Build history of the part. All positions in model axes, mm. A direction names the side the tool comes from. Round coordinates to 2 decimals unless told otherwise and drop trailing zeros. Write each loop counter-clockwise with the first axis right and the second up, starting at its lowest first coordinate (ties: lowest second). Pieces come first, ordered by that corner, then holes. Notation, with made-up numbers: (45.5, 41.25) - (92.5, 41.25) arc R15 ccw to (92.5, 55.25) - close; hole circle Ø2 at (25, 20.25). An arc over 180 degrees is marked (long way). Write each question's results on one line, items separated by ' | '.
from build123d import *

# Parameters (mm, degrees)
SKETCH_2_W                    = 30
SKETCH_2_H                    = 30
EXTRUDE_1_DEPTH               = 10
SHELL_1_T                     = -2
CUT_EXTRUDE_1_REACH           = 34.104
SKETCH_3_W                    = 28
SKETCH_3_H                    = 26
EXTRUDE_2_DEPTH               = 30
CUT_EXTRUDE_2_DEPTH           = 34.566112599
SKETCH_6_R                    = 2.375
EXTRUDE_3_DEPTH               = 1
SKETCH_7_R                    = 1
CUT_EXTRUDE_3_DEPTH           = 3
CUT_EXTRUDE_3_DRAFT           = -2
CUT_EXTRUDE_3_PROFILE_2_DEPTH = 3
CUT_EXTRUDE_3_PROFILE_2_DRAFT = -2
CUT_EXTRUDE_3_PROFILE_3_DEPTH = 3
CUT_EXTRUDE_3_PROFILE_3_DRAFT = -2
CUT_EXTRUDE_3_PROFILE_4_DEPTH = 3
CUT_EXTRUDE_3_PROFILE_4_DRAFT = -2
FILLET_2_R                    = 2
FILLET_3_R                    = 4
SKETCH_8_R                    = 1.05
CUT_EXTRUDE_4_DEPTH           = 38.710498044
CHAMFER_1_SIZE                = 1
CHAMFER_2_SIZE                = 2.001261587
CHAMFER_2_SIZE_2              = 2


with BuildPart() as part:
    # 草图2 → 凸台-拉伸1 (new body)
    with BuildSketch(Plane.XY):
        with Locations((3.057614324, -9.588661073)):
            Rectangle(SKETCH_2_W, SKETCH_2_H)
    extrude(amount=-EXTRUDE_1_DEPTH)

    # 抽壳1
    shell_1_openings = [part.faces().sort_by_distance(p)[0] for p in [
        (-11.942385676, -9.588661073, -5),
    ]]
    offset(amount=SHELL_1_T, openings=shell_1_openings, kind=Kind.INTERSECTION)

    # 草图3 → 切除-拉伸1 (cut, up to next)
    with BuildSketch(Plane.XY, mode=Mode.PRIVATE) as cut_extrude_1_sk1:
        with Locations((2.057614324, -9.588661073)):
            Rectangle(SKETCH_3_W, SKETCH_3_H)
    cut_extrude_1_tool1 = extrude(cut_extrude_1_sk1.sketch, amount=-CUT_EXTRUDE_1_REACH, mode=Mode.PRIVATE) & part.part
    add(cut_extrude_1_tool1.solids().sort_by_distance((2.057614, -9.588661, 0))[0], mode=Mode.SUBTRACT)

    # 草图4 → 凸台-拉伸2 (add)
    with BuildSketch(Plane.XZ.offset(24.588661073)):
        with BuildLine():
            Line((-11.942385676, -10), (-11.942385676, -14))
            add(Edge.make_bspline(
                [(-11.942385676, -14), (-1.471769767, -14.006598556), (8.440678476, -13.813297469), (18.057614324, -10)],
                knots=[0, 0, 0, 0, 1, 1, 1, 1], degree=3))
            Line((18.057614324, -10), (-11.942385676, -10))
        make_face()
    extrude(amount=-EXTRUDE_2_DEPTH)

    # 草图5 → 切除-拉伸2 (cut, through all)
    with BuildSketch(Plane.XY):
        with BuildLine():
            Line((6.557614324, -3.588661073), (-11.942385676, -3.588661073))
            Line((-11.942385676, -3.588661073), (-11.942385676, -15.588661073))
            Line((-11.942385676, -15.588661073), (6.557614324, -15.588661073))
            ThreePointArc((6.557614324, -15.588661073), (7.618274496, -15.149321245), (8.057614324, -14.088661073))
            Line((8.057614324, -14.088661073), (8.057614324, -5.088661073))
            ThreePointArc((8.057614324, -5.088661073), (7.618274496, -4.028000901), (6.557614324, -3.588661073))
        make_face()
    extrude(amount=-CUT_EXTRUDE_2_DEPTH, mode=Mode.SUBTRACT)

    # 草图6 → 凸台-拉伸3 (add)
    with BuildSketch(Plane.XY.offset(-8)):
        with Locations(Location((1.557614324, 0.908700453, 0), (0, 0, 180))):
            Circle(SKETCH_6_R)
        with Locations((14.057614324, 0.908700453)):
            Circle(SKETCH_6_R)
        with Locations(Location((1.557614324, -20.091299547, 0), (0, 0, 180))):
            Circle(SKETCH_6_R)
        with Locations((14.057614324, -20.091299547)):
            Circle(SKETCH_6_R)
    extrude(amount=EXTRUDE_3_DEPTH)


with BuildPart() as cut_extrude_3_tool:
    # 草图7 → 切除-拉伸3 (with draft: the straight prism first)
    with BuildSketch(Plane.XY.offset(-7)):
        with Locations((1.557614324, -20.091299547)):
            Circle(SKETCH_7_R)
    extrude(amount=-CUT_EXTRUDE_3_DEPTH)
    # 切除-拉伸3: the draft: its side faces are tilted about the plane it starts from
    cut_extrude_3_sides = [cut_extrude_3_tool.faces().sort_by_distance(p)[0] for p in [
        (0.557614324, -20.091299547, -8.5),
    ]]
    draft(cut_extrude_3_sides, Plane.XY.offset(-7), CUT_EXTRUDE_3_DRAFT)


with BuildPart() as part_1:
    add(part.part)

    # 切除-拉伸3: cut by cut_extrude_3_tool
    add(cut_extrude_3_tool.part, mode=Mode.SUBTRACT)


with BuildPart() as cut_extrude_3_profile_2_tool:
    # 草图7 → 切除-拉伸3 profile 2 (with draft: the straight prism first)
    with BuildSketch(Plane.XY.offset(-7)):
        with Locations((14.057614324, -20.091299547)):
            Circle(SKETCH_7_R)
    extrude(amount=-CUT_EXTRUDE_3_PROFILE_2_DEPTH)
    # 切除-拉伸3 profile 2: the draft: its side faces are tilted about the plane it starts from
    cut_extrude_3_profile_2_sides = [cut_extrude_3_profile_2_tool.faces().sort_by_distance(p)[0] for p in [
        (13.057614324, -20.091299547, -8.5),
    ]]
    draft(cut_extrude_3_profile_2_sides, Plane.XY.offset(-7), CUT_EXTRUDE_3_PROFILE_2_DRAFT)


with BuildPart() as part_2:
    add(part_1.part)

    # 切除-拉伸3 profile 2: cut by cut_extrude_3_profile_2_tool
    add(cut_extrude_3_profile_2_tool.part, mode=Mode.SUBTRACT)


with BuildPart() as cut_extrude_3_profile_3_tool:
    # 草图7 → 切除-拉伸3 profile 3 (with draft: the straight prism first)
    with BuildSketch(Plane.XY.offset(-7)):
        with Locations((1.557614324, 0.908700453)):
            Circle(SKETCH_7_R)
    extrude(amount=-CUT_EXTRUDE_3_PROFILE_3_DEPTH)
    # 切除-拉伸3 profile 3: the draft: its side faces are tilted about the plane it starts from
    cut_extrude_3_profile_3_sides = [cut_extrude_3_profile_3_tool.faces().sort_by_distance(p)[0] for p in [
        (0.557614324, 0.908700453, -8.5),
    ]]
    draft(cut_extrude_3_profile_3_sides, Plane.XY.offset(-7), CUT_EXTRUDE_3_PROFILE_3_DRAFT)


with BuildPart() as part_3:
    add(part_2.part)

    # 切除-拉伸3 profile 3: cut by cut_extrude_3_profile_3_tool
    add(cut_extrude_3_profile_3_tool.part, mode=Mode.SUBTRACT)


with BuildPart() as cut_extrude_3_profile_4_tool:
    # 草图7 → 切除-拉伸3 profile 4 (with draft: the straight prism first)
    with BuildSketch(Plane.XY.offset(-7)):
        with Locations((14.057614324, 0.908700453)):
            Circle(SKETCH_7_R)
    extrude(amount=-CUT_EXTRUDE_3_PROFILE_4_DEPTH)
    # 切除-拉伸3 profile 4: the draft: its side faces are tilted about the plane it starts from
    cut_extrude_3_profile_4_sides = [cut_extrude_3_profile_4_tool.faces().sort_by_distance(p)[0] for p in [
        (13.057614324, 0.908700453, -8.5),
    ]]
    draft(cut_extrude_3_profile_4_sides, Plane.XY.offset(-7), CUT_EXTRUDE_3_PROFILE_4_DRAFT)


with BuildPart() as part_4:
    add(part_3.part)

    # 切除-拉伸3 profile 4: cut by cut_extrude_3_profile_4_tool
    add(cut_extrude_3_profile_4_tool.part, mode=Mode.SUBTRACT)

    # 圆角2
    fillet_2_edges = [part_4.edges().sort_by_distance(p)[0] for p in [
        (16.057614324, 3.411338927, -4),
        (16.057614324, -22.588661073, -4),
    ]]
    fillet(fillet_2_edges, radius=FILLET_2_R)

    # 圆角3
    fillet_3_edges = [part_4.edges().sort_by_distance(p)[0] for p in [
        (18.057614324, -24.588661073, -5),
        (18.057614324, 5.411338927, -5),
    ]]
    fillet(fillet_3_edges, radius=FILLET_3_R)

    # 草图8 → 切除-拉伸4 (cut, through all)
    with BuildSketch(Plane(origin=(0, 5.411338927, 0), x_dir=(1, 0, 0), z_dir=(0, 1, 0))):
        with Locations(Location((8.874069652, 2.5, 0), (0, 0, 180))):
            Circle(SKETCH_8_R)
    extrude(amount=-CUT_EXTRUDE_4_DEPTH, mode=Mode.SUBTRACT)

    # 倒角1
    chamfer_1_edges = [part_4.edges().sort_by_distance(p)[0] for p in [
        (9.924069652, -24.588661073, -2.5),
        (9.924069652, 5.411338927, -2.5),
    ]]
    chamfer(chamfer_1_edges, length=CHAMFER_1_SIZE)

    # 倒角2
    # the kernel refuses this chamfer: 2.001261587, 2 mm, written as the material it takes off along each edge
    with BuildSketch(Plane(origin=(-11.942385676, -8.735358117, -14), x_dir=(0.9999994656090836, 0, 0.0010338189141659818), z_dir=(0, 1, 0))) as chamfer_2_piece_1:
        with BuildLine():
            Line((1.996680257, 0), (CHAMFER_2_SIZE * 0.00103381891429, -CHAMFER_2_SIZE * 0.99999946573))
            Line((CHAMFER_2_SIZE * 0.00103381891429, -CHAMFER_2_SIZE * 0.99999946573), (0, 0))
            ThreePointArc((0, 0), (1.026596764, 0.000946618), (1.996680257, 0))
        make_face()
    extrude(amount=19.293394088, mode=Mode.SUBTRACT)
    with BuildSketch(Plane(origin=(-11.942385676, -29.732118676, -14), x_dir=(0.99999946423231, 0, 0.001035149792544402), z_dir=(0, 1, 0))) as chamfer_2_piece_2:
        with BuildLine():
            Line((1.997932911, 0), (CHAMFER_2_SIZE_2 * 0.00103514979254, -CHAMFER_2_SIZE_2 * 0.999999464232))
            Line((CHAMFER_2_SIZE_2 * 0.00103514979254, -CHAMFER_2_SIZE_2 * 0.999999464232), (0, 0))
            ThreePointArc((0, 0), (1.027240915, 0.000948024), (1.997932911, 0))
        make_face()
    extrude(amount=19.286915207, mode=Mode.SUBTRACT)


solid = part_4.part
(1) Drill centre lines: probe 1 along Y at (x, z) = (-4.5, -10.75); probe 2 along X at (y, z) = (-2, -4.5); probe 3 along Z at (x, y) = (8, -19). Where is each one in solid material? Low to high. Write a range as [from, to].
Worked answers:
probe 1: y = [-24.59, -15.59], [-3.59, 5.41] | probe 2: x = [16.06, 18.06] | probe 3: z = [-12.79, -8]
(2) Flat gauge pins, fed straight in: pin 1 Ø1.4 at (x, y) = (1.5, -20.5) entering from +Z; pin 2 Ø3 at (x, y) = (10, -12.5) entering from +Z; pin 3 Ø1.7 at (x, z) = (8.87, -2.5) entering from -Y; pin 4 Ø1 at (y, z) = (-11, -10.5) entering from -X. Where does each tip first touch, or does it go through?
Worked answers:
pin 1: stops at z = -7 | pin 2: stops at z = -8 | pin 3: passes through | pin 4: stops at x = 8.06
(3) Slice it at A-A, the plane z = -2.5. Write the cut outline in (x, y).
Worked answers:
outline: (-11.94, -24.59) - (6.82, -24.59) - (7.82, -23.59) - (7.82, -22.59) - (-11.94, -22.59) - close; (-11.94, 3.41) - (7.82, 3.41) - (7.82, 4.41) - (6.82, 5.41) - (-11.94, 5.41) - close; (9.92, -23.59) - (10.92, -24.59) - (14.06, -24.59) arc R4 ccw to (18.06, -20.59) - (18.06, 1.41) arc R4 ccw to (14.06, 5.41) - (10.92, 5.41) - (9.92, 4.41) - (9.92, 3.41) - (14.06, 3.41) arc R2 cw to (16.06, 1.41) - (16.06, -20.59) arc R2 cw to (14.06, -22.59) - (9.92, -22.59) - close
(4) Slice it at C-C, the plane x = 9.5. State how many separate pieces and enclosed holes the cut face has, and give its area (3 significant figures).
Worked answers:
separate pieces: 3 | enclosed holes: 0 | area: 158 mm2
(5) Two-plate mould, pull along Y, no slides. Class faces 4 (the flat face through (16.3, -9.5, 0)), 5 (the flat face through (1, -24.589, -7)), 6 (the flat face through (8, -4, -8)): released by +Y, released by -Y, zero draft, split by the parting line, or undercut.
Worked answers:
face 4: zero draft | face 5: released by -Y | face 6: undercut
(6) Tool access for faces 1 (the flat face through (-10.93, -20.15, -13.01)), 2 (the flat face through (-3, -15.589, -11)), 3 (the cylindrical face through (0.281, -22.094, -7.507)): list every direction of +Z, -Z, +X, -X, +Y, -Y with a clear straight run to the whole face (end or side of a thin tool).
Worked answers:
face 1: -Z, -X, +Y, -Y | face 2: +Z, -Z, -X | face 3: +Z
(7) Slice it at B-B, the plane z = -5. Write the cut outline in (x, y).
Worked answers:
outline: (-11.94, -24.59) - (14.06, -24.59) arc R4 ccw to (18.06, -20.59) - (18.06, 1.41) arc R4 ccw to (14.06, 5.41) - (-11.94, 5.41) - (-11.94, 3.41) - (14.06, 3.41) arc R2 cw to (16.06, 1.41) - (16.06, -20.59) arc R2 cw to (14.06, -22.59) - (-11.94, -22.59) - close
